Input: part model. Units: mm. Frame: model coordinates. Give positions to 0.01 mm unless a question says otherwise; leave off trailing zeros. Write each loop counter-clockwise with the first axis right and the second up, starting at its lowest first coordinate (ties: lowest second). Pieces come first, ordered by that corner, then holes. Notation, with made-up numbers: (-3.75, 65) - (29.25, 65) arc R16 cw to (29.25, 85) - close; hole circle Ø11 at (-38, -4). An arc over 180 degrees is marked (long way). Use a Markdown table: item, result. Add a question column.
1. Section query B-B, the plane y = -29. Return loops of the section in (x, z).
2. Material intervals for probe 1 along Y at (x, z) = (13.4, -11.5); probe 2 along Y at (x, z) = (13.95, -19.5); probe 3 along Z at (x, y) = (14.05, -37.75), sorted ascending.
3. Section query C-C, the plane x = 14. Return loops of the section in (y, z), plus the area to 3 significant figures.
4. Section query D-D, the plane y = -20. Return loops of the section in (x, z), plus the area to 3 significant figures.
5. Section query A-A, the plane z = -11.5. Return loops of the section in (x, y), plus the area to 3 significant figures.
6. Pin query (flat end, axial travel): pin 1 (6 mm diameter, centred on y = -29, z = -19.5, fed in from +X). Return the tip coordinate at first contact, or that it passes through.
```python
from build123d import *

# Parameters (mm, degrees)
THRUST_PLATE_BLANK_SKETCH_W      = 2
THRUST_PLATE_BLANK_SKETCH_H      = 24
THRUST_PLATE_BLANK_DEPTH         = 24
SCREW_RUNNING_CLEARANCE_SKETCH_R = 3.25
SCREW_RUNNING_CLEARANCE_DEPTH    = 2.2
M3_PLATE_CLEARANCE_1_SKETCH_R    = 1.7
M3_PLATE_CLEARANCE_1_DEPTH       = 2.2
M3_PLATE_CLEARANCE_2_SKETCH_R    = 1.7
M3_PLATE_CLEARANCE_2_DEPTH       = 2.2


with BuildPart() as part:
    # Thrust plate blank sketch → Thrust plate blank (new body)
    with BuildSketch(Plane.XY.offset(-31.5)):
        with Locations((14, -29)):
            Rectangle(THRUST_PLATE_BLANK_SKETCH_W, THRUST_PLATE_BLANK_SKETCH_H)
    extrude(amount=THRUST_PLATE_BLANK_DEPTH)

    # Screw running clearance sketch → Screw running clearance (cut)
    with BuildSketch(Plane(origin=(12.9, 0, 0), x_dir=(0, 0, -1), z_dir=(1, 0, 0))):
        with Locations(Location((19.5, -29, 0), (0, 0, 180))):
            Circle(SCREW_RUNNING_CLEARANCE_SKETCH_R)
    extrude(amount=SCREW_RUNNING_CLEARANCE_DEPTH, mode=Mode.SUBTRACT)

    # M3 plate clearance 1 sketch → M3 plate clearance 1 (cut)
    with BuildSketch(Plane(origin=(12.9, 0, 0), x_dir=(0, 0, -1), z_dir=(1, 0, 0))):
        with Locations(Location((11.5, -38, 0), (0, 0, 180))):
            Circle(M3_PLATE_CLEARANCE_1_SKETCH_R)
    extrude(amount=M3_PLATE_CLEARANCE_1_DEPTH, mode=Mode.SUBTRACT)

    # M3 plate clearance 2 sketch → M3 plate clearance 2 (cut)
    with BuildSketch(Plane(origin=(12.9, 0, 0), x_dir=(0, 0, -1), z_dir=(1, 0, 0))):
        with Locations(Location((11.5, -20, 0), (0, 0, 180))):
            Circle(M3_PLATE_CLEARANCE_2_SKETCH_R)
    extrude(amount=M3_PLATE_CLEARANCE_2_DEPTH, mode=Mode.SUBTRACT)


solid = part.part
```
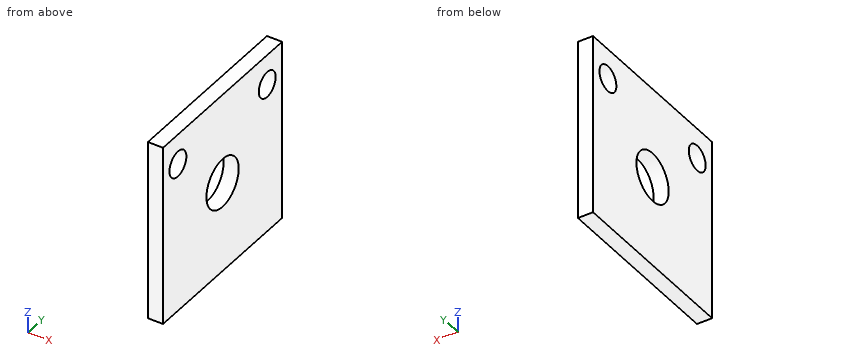
Result sheet:
| question | item | result |
|---|---|---|
| 1 | outline | (13, -31.5) - (15, -31.5) - (15, -22.75) - (13, -22.75) - close; (13, -16.25) - (15, -16.25) - (15, -7.5) - (13, -7.5) - close |
| 2 | probe 1 | y = -41 to -39.7, -36.3 to -21.7, -18.3 to -17 |
| 2 | probe 2 | y = -41 to -32.25, -25.75 to -17 |
| 2 | probe 3 | z = -31.5 to -13.18, -9.82 to -7.5 |
| 3 | outline | (-41, -31.5) - (-17, -31.5) - (-17, -7.5) - (-41, -7.5) - close; hole circle Ø3.4 at (-38, -11.5); hole circle Ø6.5 at (-29, -19.5); hole circle Ø3.4 at (-20, -11.5) |
| 3 | area | 525 mm² |
| 4 | outline | (13, -31.5) - (15, -31.5) - (15, -13.2) - (13, -13.2) - close; (13, -9.8) - (15, -9.8) - (15, -7.5) - (13, -7.5) - close |
| 4 | area | 41.2 mm² |
| 5 | outline | (13, -41) - (15, -41) - (15, -39.7) - (13, -39.7) - close; (13, -36.3) - (15, -36.3) - (15, -21.7) - (13, -21.7) - close; (13, -18.3) - (15, -18.3) - (15, -17) - (13, -17) - close |
| 5 | area | 34.4 mm² |
| 6 | pin 1 | passes through |
